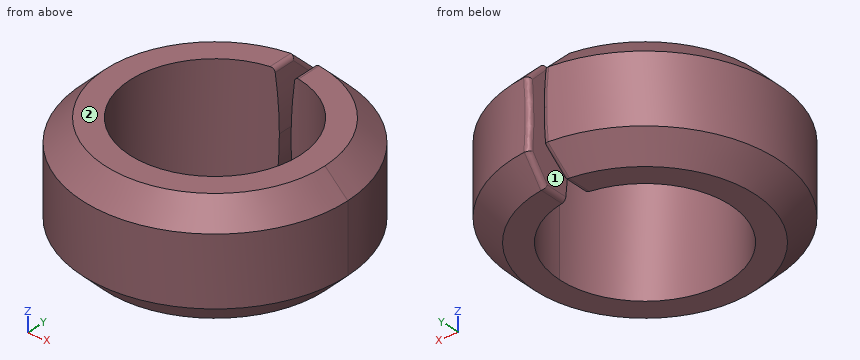
from build123d import *

# Parameters (mm, degrees)
F1_DEPTH = 19.05
F2_SIZE  = 3.81
F4_DEPTH = 25.4
F5_R     = 0.762


with BuildPart() as f1:
    # F0 (on Top) → F1 (new body)
    with BuildSketch(Plane.XY):
        with BuildLine():
            ThreePointArc((0.8676202269, 14.2685876747), (10.4102819289, 9.7964988261), (14.2949417309, 0))
            ThreePointArc((14.2949417309, 0), (-9.7964988261, -10.4102819289), (-0.8676202269, 14.2685876747))
            Line((-0.8676202269, 14.2685876747), (-0.8676202269, 22.2080584505))
            ThreePointArc((-0.8676202269, 22.2080584505), (-15.4056445087, -16.019261602), (22.225, 0))
            ThreePointArc((22.225, 0), (16.019261602, 15.4056445087), (0.8676202269, 22.2080584505))
            Line((0.8676202269, 22.2080584505), (0.8676202269, 14.2685876747))
        make_face()
    extrude(amount=F1_DEPTH)

    # F2
    f2_edges = [f1.edges().sort_by_distance(p)[0] for p in [
        (-15.405645, -16.019262, 19.05),
        (-15.405645, -16.019262, 0),
    ]]
    chamfer(f2_edges, length=F2_SIZE)

    # F3 (on Front) → F4 (cut)
    with BuildSketch(Plane.XZ):
        with BuildLine():
            ThreePointArc((2.6717553826, -5.5055550528), (0.9808079105, 9.7828422745), (2.9202771279, 25.0417038096))
            Line((2.9202771279, 25.0417038096), (-2.9202771279, 25.0417038096))
            ThreePointArc((-2.9202771279, 25.0417038096), (-1.465879157, 17.2066583018), (-0.9786513266, 9.2526768707))
            ThreePointArc((-0.9786513266, 9.2526768707), (-1.4033109655, 1.8251602795), (-2.6717553826, -5.5055550528))
            Line((-2.6717553826, -5.5055550528), (2.6717553826, -5.5055550528))
        make_face()
    extrude(amount=-F4_DEPTH, mode=Mode.SUBTRACT)

    # F5
    f5_edges = [f1.edges().sort_by_distance(p)[0] for p in [
        (-1.45887, 20.2631, 17.149451),
        (1.45887, 20.2631, 17.149451),
        (-0.979225, 22.203417, 9.526057),
        (0.979225, 22.203417, 9.526057),
        (1.719324, 16.262865, 19.05),
        (-1.719324, 16.262865, 19.05),
        (-1.394665, 20.267988, 1.900916),
        (-1.638853, 16.271309, 0),
        (1.394665, 20.267988, 1.900916),
        (1.638853, 16.271309, 0),
    ]]
    fillet(f5_edges, radius=F5_R)


solid = f1.part
Geometry: final body of the model. Coordinates: model frame, mm. Face numbers are marked on the shaded views. A direction names the side the tool comes from. Round coordinates to 2 decimals unless told otherwise and drop trailing zeros. Order: outer loops, then holes, each group sorted by start corner. A loop starts at its lowest first (then second) coordinate and runs counter-clockwise, first axis right, second up. Notation, with made-up numbers: (35.5, 87) - (53.5, 87) arc R24 cw to (53.5, 123) - close; hole circle Ø7 at (50, -11). An arc over 180 degrees is marked (long way). Write each question's results on one line, items separated by ' | '.
Item 1: Material intervals for line 1 along X through (y, z) = (0.5, 5.25); line 2 along Y through (x, z) = (0, 5) (3 decimals); line 3 along X through (y, z) = (14.5, 11.75), sorted ascending. Write a range as [from, to].
Completed:
line 1: [-22.22, -14.29], [14.29, 22.22] | line 2: [-22.225, -14.295] | line 3: [-16.84, -1.03], [1.03, 16.84]
Item 2: Reachability of the marked faces 1 and 2 from +Z, -Z, +X, -X, +Y, -Y: full face, straight path, thin tool, end or side. Return the list, or none.
Completed:
face 1: +Y | face 2: +Z, +X, -X, +Y, -Y
Item 3: Section A-A, the plane x = 0. Return the cut outline in (y, z) (3 decimals), and give its area (3 significant figures).
Completed:
outline: (-22.225, 3.81) - (-18.415, 0) - (-14.295, 0) - (-14.295, 19.05) - (-18.415, 19.05) - (-22.225, 15.24) - close | area: 137 mm^2
Item 4: First-contact query: pin 1 Ø3 at (x, z) = (-13.5, 14) entering from -Y; pin 2 Ø8 at (x, z) = (13, 8.5) entering from -Y; pin 3 Ø2 at (x, z) = (0, 17) entering from -Y (3 decimals). Flat tips, straight axial feed; report the tip coordinate or a pass-through.
Completed:
pin 1: y = -18.71 | pin 2: y = -20.32 | pin 3: y = -21.465
